Work out the finished part from the listing and answer in its coordinate system (mm). Round coordinates to 2 decimals unless told otherwise and drop trailing zeros. Order: outer loops, then holes, each group sorted by start corner. A loop starts at its lowest first (then second) coordinate and runs counter-clockwise, first axis right, second up. Notation, with made-up numbers: M -36,6.5 L -8,6.5 A23 ccw -8,23.5 Z; hole C 38,60 d5. An arc over 180 degrees is marked long. Return JSON: item names as keys, results as strings.
from build123d import *

# Parameters (mm, degrees)
F2_R     = 3.25
F3_DEPTH = 29.531188
F4_R     = 4.85
F5_DEPTH = 25


with BuildPart() as f1:
    # F0 (on Front) → F1 (revolve)
    with BuildSketch(Plane.XZ):
        with BuildLine():
            Line((0, -11.765188), (0, 0))
            Line((0, 0), (-5, 0))
            Line((-5, 0), (-5, 10.649866))
            ThreePointArc((-5, 10.649866), (-11.482973, -2.561442), (0, -11.765188))
        make_face()
        with BuildLine():
            Line((-5, 0), (0, 0))
            Line((0, 0), (0, 11.765188))
            ThreePointArc((0, 11.765188), (-2.561442, 11.482973), (-5, 10.649866))
            Line((-5, 10.649866), (-5, 0))
        make_face()
        with BuildLine():
            ThreePointArc((-5, 10.649866), (-2.561442, 11.482973), (0, 11.765188))
            Line((0, 11.765188), (0, 17.765))
            Line((0, 17.765), (-5, 17.765))
            Line((-5, 17.765), (-5, 10.649866))
        make_face()
    revolve(axis=Axis((0, 0, 8.8825), (0, 0, 1)))

    # F2 (on face) → F3 (cut, through all)
    with BuildSketch(Plane.XY.offset(17.765)):
        Circle(F2_R)
    extrude(amount=-F3_DEPTH, mode=Mode.SUBTRACT)

    # F4 (on Top) → F5 (cut)
    with BuildSketch(Plane.XY):
        Circle(F4_R)
    extrude(amount=-F5_DEPTH, mode=Mode.SUBTRACT)


solid = f1.part
Item 1: The mould has two halves that part along Y. Classify faces 1 (the cylindrical face through (-2.579, -1.978, 9.007)), 2 (the flat face through (3.3, 1, 17.765)), 3 (the cylindrical face through (1.08, 4.88, 14.16)): pulls with the +Y half, pulls with the -Y half, needs draft (parallel to the pull), parting line crosses it, or undercut.
Output:
{"face 1": "undercut", "face 2": "needs draft", "face 3": "parting line crosses it"}
Item 2: Consider line 1 along X through (y, z) = (0.25, -0.25); line 2 along Y through (x, z) = (0, 12.5); line 3 along X through (y, z) = (0, -2.5). Determine where each line is inside the solid, lowest interval first. Write a range as [from, to].
Output:
{"line 1": "x = [-11.76, -4.84], [4.84, 11.76]", "line 2": "y = [-5, -3.25], [3.25, 5]", "line 3": "x = [-11.5, -4.85], [4.85, 11.5]"}
Item 3: Each of these flat-tipped pins is pushed along its axis until it touches: pin 1 (3 mm diameter, centred on x = 4, y = 6.5, fed in from +Z); pin 2 (8 mm diameter, centred on y = -5.5, z = -1, fed in from +X); pin 3 (10 mm diameter, centred on x = 1, z = 8, fed in from -Y). Where does it stop, or does it pass through?
Output:
{"pin 1": "stops at z = 10.04", "pin 2": "stops at x = 11.66", "pin 3": "stops at y = -11.36"}
Item 4: Find section A-A (z = 15.25). Determine the outline of the cut face in (x, y).
Output:
{"outline": "C 0,0 d10; hole C 0,0 d6.5"}
